Print and shaded views of the part. All mm, measured from the part's lowest x, y and z. A direction names the side the tool comes from. Round coordinates to 2 decimals unless told otherwise and drop trailing zeros. Order: outer loops, then holes, each group sorted by start corner. A loop starts at its lowest first (then second) coordinate and runs counter-clockwise, first axis right, second up. Notation, with made-up numbers: (29, -29.5) - (81, -29.5) arc R25 cw to (81, 9.5) - close; hole circle Ø5 at (28.25, 24). An arc over 180 degrees is marked (long way). Return JSON: item names as keys, results as strings. Group by question number.
Item 1: Drop flat-ended pins along their axis: pin 1 (4 mm diameter, centred on x = 18, z = 15.5, fed in from +Y); pin 2 (2.5 mm diameter, centred on x = 38, z = 14.5, fed in from +Y); pin 3 (5 mm diameter, centred on x = 31, y = 14.5, fed in from -Z). Give the stop position or say it passes through.
Item 2: Saw through at D-D on y = 19.5. List the corners of the cut face in (x, z).
Item 3: Saw through at C-C on x = 52. List the corners of the cut face in (y, z).
Item 4: Saw through at A-A on y = 23.8. State how many separate pieces and enclosed holes the cut face has, and give its area (3 significant figures).
Item 5: Two-plate mould, pull along Z, no slides. Class the marked faces 3, 4, 5 and 6: released by +Z, released by -Z, zero draft, split by the parting line, or undercut.
Item 6: Tool access for the marked faces 1 and 2: list every direction of +Z, -Z, +X, -X, +Y, -Y with a clear straight run to the whole face (end or side of a thin tool).
Item 7: Probe probe 1 along Z at (x, y) = (35, 10); probe 2 along Y at (x, z) = (10.25, 28.55); probe 3 along Y at (x, z) = (68, 6). List the from-to ranges inside material, lowest first.
Item 8: Saw through at B-B on z = 21.5. List the corners of the cut face in (x, y).
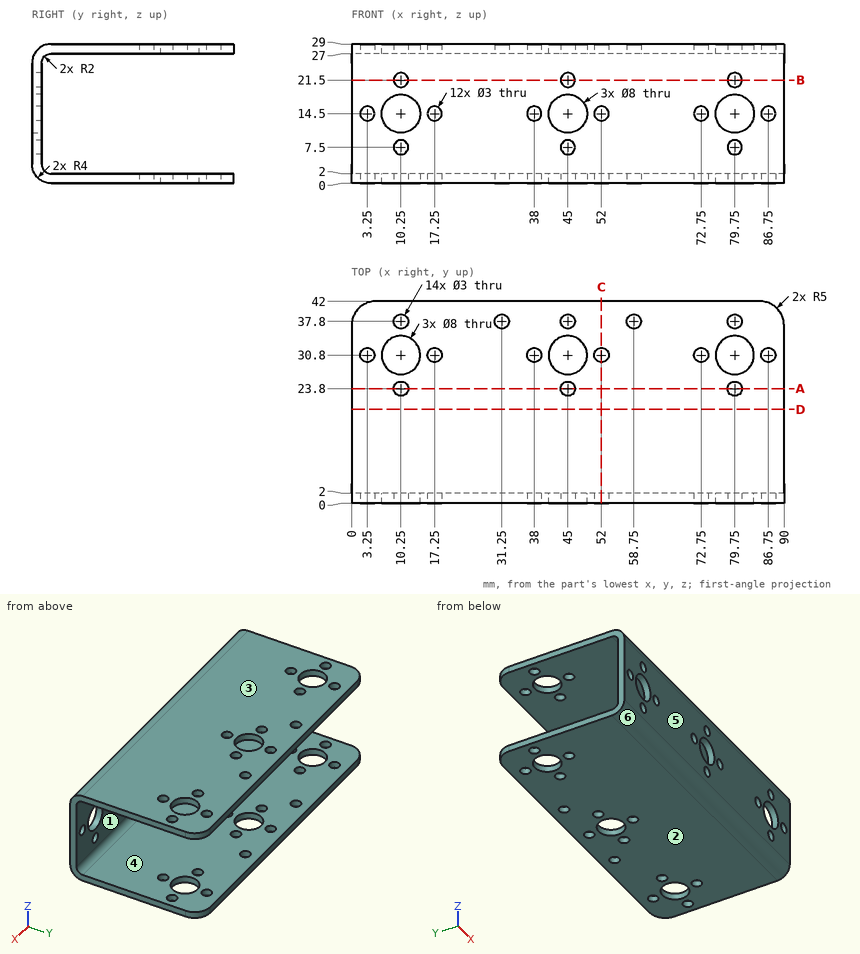
Filled in:
{
 "1": {"pin 1": "stops at y = 2", "pin 2": "passes through", "pin 3": "stops at z = 0"},
 "2": {"outline": "(0, 0) - (90, 0) - (90, 2) - (0, 2) - close; (0, 27) - (90, 27) - (90, 29) - (0, 29) - close"},
 "3": {"outline": "(0, 4) arc R4 ccw to (4, 0) - (29.3, 0) - (29.3, 2) - (4, 2) arc R2 cw to (2, 4) - (2, 13) - (0, 13) - close; (0, 16) - (2, 16) - (2, 25) arc R2 cw to (4, 27) - (29.3, 27) - (29.3, 29) - (4, 29) arc R4 ccw to (0, 25) - close; (32.3, 0) - (42, 0) - (42, 2) - (32.3, 2) - close; (32.3, 27) - (42, 27) - (42, 29) - (32.3, 29) - close"},
 "4": {"separate pieces": "8", "enclosed holes": "0", "area": "324 mm^2"},
 "5": {"face 3": "released by +Z", "face 4": "undercut", "face 5": "zero draft", "face 6": "released by -Z"},
 "6": {"face 1": "+X, -X, +Y", "face 2": "-Z, +X, -X, +Y, -Y"},
 "7": {"probe 1": "z = 0 to 2, 27 to 29", "probe 2": "y = 2.16 to 22.3, 25.3 to 26.8, 34.8 to 36.3, 39.3 to 42", "probe 3": "y = 0 to 2"},
 "8": {"outline": "(0, 0) - (8.75, 0) - (8.75, 2) - (0, 2) - close; (11.75, 0) - (43.5, 0) - (43.5, 2) - (11.75, 2) - close; (46.5, 0) - (78.25, 0) - (78.25, 2) - (46.5, 2) - close; (81.25, 0) - (90, 0) - (90, 2) - (81.25, 2) - close"}
}
